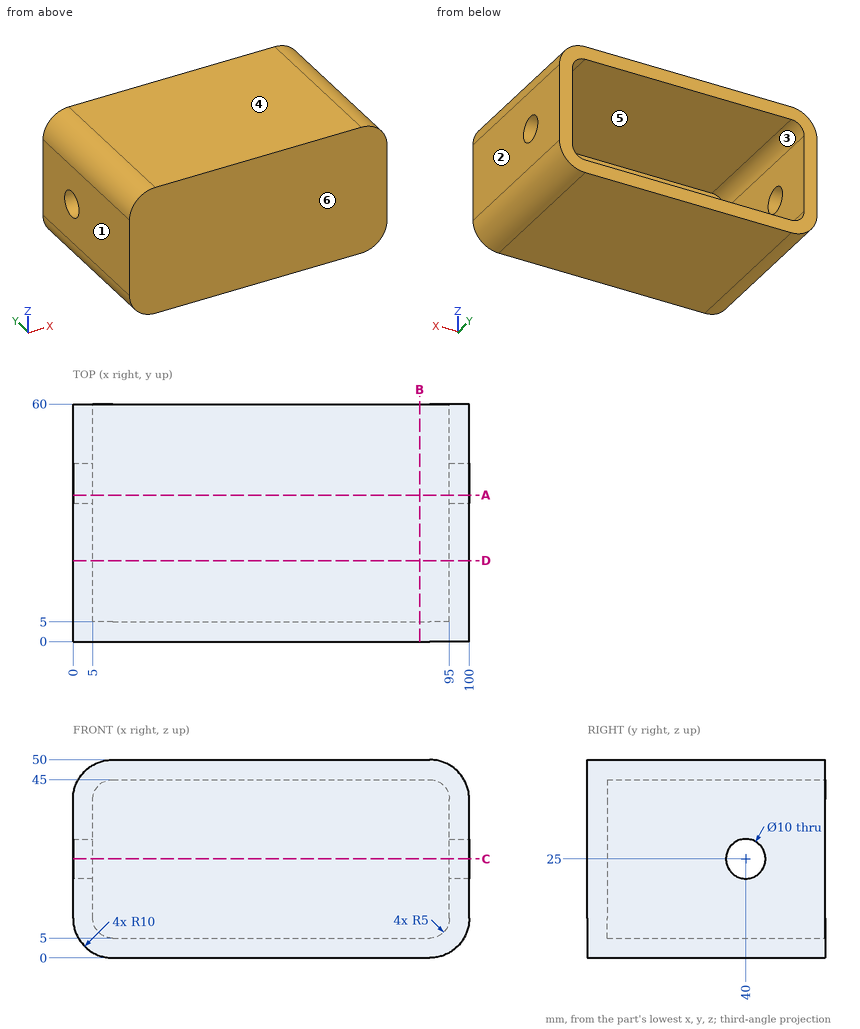
Check sheet for the drawn part. Datum: minimum x, y, z corner. Units: mm. A direction names the side the tool comes from. Coordinates: 2 decimals unless noted, no trailing zeros. Loops run counter-clockwise (first coordinate to the right, second up) from the corner with the lowest first, then second, coordinate; pieces in that order, holes last. Notation, with made-up numbers: (-8.75, -31.75) -> (14.25, -31.75) arc R24 cw to (14.25, -10.75) -> close; hole circle Ø11 at (27.5, 29.25). An arc over 180 degrees is marked (long way). Answer as a JSON object with one key per item and string values. Group by question number.
Item 1: Mould release check, pull along X, two halves, no side actions. Record for the marked faces 1, 2, 3 and 4: +X half, -X half, draft (parallel to the pull), parting line (faces both ways), or undercut.
Item 2: Scan lines: probe 1 along X at (y, z) = (54, 30); probe 2 along Z at (x, y) = (32, 53); probe 3 along Y at (x, z) = (97.35, 25). Record each from-to range of solid material in increasing order.
Item 3: Depth check by flat-ended pin: pin 1 (1 mm diameter, centred on x = 76, z = 33, fed in from +Y); pin 2 (1.5 mm diameter, centred on x = 37, y = 23.5, fed in from -Z); pin 3 (9 mm diameter, centred on y = 40, z = 25, fed in from -X). Enter the tip coordinate at first touch or a pass-through.
Item 4: Sectioned sample at D-D on y = 20.5. Record the boundary of the cut face in (x, z), plus the area to 3 significant figures.
Item 5: Tool access check on the marked faces 5 and 6. Record the directions out of +Z, -Z, +X, -X, +Y, -Y that give a thin tool (end or side, any length) a straight path to the whole face; none if there is none.
Item 6: Sectioned sample at B-B on x = 87.5. Record the boundary of the cut face in (y, z).
Item 7: Sectioned sample at A-A on y = 37. Record the boundary of the cut face in (x, z).
Item 8: Sectioned sample at C-C on z = 25. Record the boundary of the cut face in (x, y).
Evaluation:
{
 "1": {"face 1": "-X half", "face 2": "+X half", "face 3": "undercut", "face 4": "draft"},
 "2": {"probe 1": "x = 0 to 5, 95 to 100", "probe 2": "z = 0 to 5, 45 to 50", "probe 3": "y = 0 to 35, 45 to 60"},
 "3": {"pin 1": "stops at y = 5", "pin 2": "stops at z = 0", "pin 3": "passes through"},
 "4": {"outline": "(0, 10) arc R10 ccw to (10, 0) -> (90, 0) arc R10 ccw to (100, 10) -> (100, 40) arc R10 ccw to (90, 50) -> (10, 50) arc R10 ccw to (0, 40) -> close; hole (5, 10) arc R5 ccw to (10, 5) -> (90, 5) arc R5 ccw to (95, 10) -> (95, 40) arc R5 ccw to (90, 45) -> (10, 45) arc R5 ccw to (5, 40) -> close", "area": "1,340 mm²"},
 "5": {"face 5": "+Y", "face 6": "+Z, -Z, +X, -X, -Y"},
 "6": {"outline": "(0, 0) -> (60, 0) -> (60, 5) -> (5, 5) -> (5, 45) -> (60, 45) -> (60, 50) -> (0, 50) -> close"},
 "7": {"outline": "(0, 10) arc R10 ccw to (10, 0) -> (90, 0) arc R10 ccw to (100, 10) -> (100, 21) -> (95, 21) -> (95, 10) arc R5 cw to (90, 5) -> (10, 5) arc R5 cw to (5, 10) -> (5, 21) -> (0, 21) -> close; (0, 29) -> (5, 29) -> (5, 40) arc R5 cw to (10, 45) -> (90, 45) arc R5 cw to (95, 40) -> (95, 29) -> (100, 29) -> (100, 40) arc R10 ccw to (90, 50) -> (10, 50) arc R10 ccw to (0, 40) -> close"},
 "8": {"outline": "(0, 0) -> (100, 0) -> (100, 35) -> (95, 35) -> (95, 5) -> (5, 5) -> (5, 35) -> (0, 35) -> close; (0, 45) -> (5, 45) -> (5, 60) -> (0, 60) -> close; (95, 45) -> (100, 45) -> (100, 60) -> (95, 60) -> close"}
}
